from build123d import *

# Parameters (mm, degrees)
SKETCH1_R           = 47.625
BOSS_EXTRUDE1_DEPTH = 19.05
CUT_EXTRUDE1_DEPTH  = 70.9941694
CIRPATTERN1_COUNT   = 10
CUT_EXTRUDE2_DEPTH  = 15.24
SKETCH5_R           = 4.064
CUT_EXTRUDE3_DEPTH  = 70.054607739
CUT_EXTRUDE4_DEPTH  = 70.9941694


with BuildPart() as part:
    # Sketch1 → Boss-Extrude1 (new body)
    with BuildSketch(Plane(origin=(0, 0, 0), x_dir=(1, 0, 0), z_dir=(0, 1, 0))):
        with Locations(Location((0, 0, 0), (0, 0, 90))):
            Circle(SKETCH1_R)
    extrude(amount=BOSS_EXTRUDE1_DEPTH)

    # Sketch3 → Cut-Extrude1 (cut, symmetric)
    with BuildSketch(Plane(origin=(0, 19.05, 0), x_dir=(1, 0, 0), z_dir=(0, 1, 0))):
        with BuildLine():
            Line((0, 47.625), (0, 34.925))
            ThreePointArc((0, 34.925), (5.463473692, 34.495015295), (10.792418529, 33.215648832))
            Line((10.792418529, 33.215648832), (14.716934357, 45.294066589))
            ThreePointArc((14.716934357, 45.294066589), (7.450191398, 47.038657221), (0, 47.625))
        make_face()
    cut_extrude1 = extrude(amount=CUT_EXTRUDE1_DEPTH, both=True, mode=Mode.SUBTRACT)

    # CirPattern1: Cut-Extrude1 ×10 about axis
    cirpattern1_axis = Axis((0, 0, 0), (0, 1, 0))
    for i in range(1, CIRPATTERN1_COUNT):
        add(cut_extrude1.rotate(cirpattern1_axis, i * 360 / CIRPATTERN1_COUNT), mode=Mode.SUBTRACT)

    # Sketch4 → Cut-Extrude2 (cut)
    with BuildSketch(Plane(origin=(0, 19.05, 0), x_dir=(1, 0, 0), z_dir=(0, 1, 0))):
        Polygon((-3.519527241, 6.096), (3.519527241, 6.096), (7.039054482, 0), (3.519527241, -6.096), (-3.519527241, -6.096), (-7.039054482, 0), align=None)
    extrude(amount=-CUT_EXTRUDE2_DEPTH, mode=Mode.SUBTRACT)

    # Sketch5 → Cut-Extrude3 (cut, through all)
    with BuildSketch(Plane(origin=(0, 3.81, 0), x_dir=(1, 0, 0), z_dir=(0, 1, 0))):
        with Locations(Location((0, 0, 0), (0, 0, 270))):
            Circle(SKETCH5_R)
    extrude(amount=-CUT_EXTRUDE3_DEPTH, mode=Mode.SUBTRACT)

    # Sketch6 → Cut-Extrude4 (cut, through all)
    with BuildSketch(Plane(origin=(0, 19.05, 0), x_dir=(1, 0, 0), z_dir=(0, 1, 0))):
        with BuildLine():
            ThreePointArc((-11.225320151, 11.225320151), (-6.075099489, 14.666587579), (0, 15.875))
            Line((0, 15.875), (0, 27.94))
            ThreePointArc((0, 27.94), (-10.6921751, 25.813194138), (-19.756563466, 19.756563466))
            Line((-19.756563466, 19.756563466), (-11.225320151, 11.225320151))
        make_face()
        with BuildLine():
            Line((19.756563466, 19.756563466), (11.225320151, 11.225320151))
            ThreePointArc((11.225320151, 11.225320151), (14.666587579, 6.075099489), (15.875, 0))
            Line((15.875, 0), (27.94, 0))
            ThreePointArc((27.94, 0), (25.813194138, 10.6921751), (19.756563466, 19.756563466))
        make_face()
        with BuildLine():
            Line((19.756563466, -19.756563466), (11.225320151, -11.225320151))
            ThreePointArc((11.225320151, -11.225320151), (6.075099489, -14.666587579), (0, -15.875))
            Line((0, -15.875), (0, -27.94))
            ThreePointArc((0, -27.94), (10.6921751, -25.813194138), (19.756563466, -19.756563466))
        make_face()
        with BuildLine():
            Line((-19.756563466, -19.756563466), (-11.225320151, -11.225320151))
            ThreePointArc((-11.225320151, -11.225320151), (-14.666587579, -6.075099489), (-15.875, 0))
            Line((-15.875, 0), (-27.94, 0))
            ThreePointArc((-27.94, 0), (-25.813194138, -10.6921751), (-19.756563466, -19.756563466))
        make_face()
    extrude(amount=-CUT_EXTRUDE4_DEPTH, mode=Mode.SUBTRACT)


solid = part.part
Geometry: final body of the model. Coordinates: model frame, mm. A direction names the side the tool comes from. Coordinates: 2 decimals unless noted, no trailing zeros. Order: outer loops, then holes, each group sorted by start corner. A loop starts at its lowest first (then second) coordinate and runs counter-clockwise, first axis right, second up.
1) Section A-A (x = -17). Return loops of the section in (y, z).
Result sheet:
outline: (0, -30.51) - (19.05, -30.51) - (19.05, -22.17) - (0, -22.17) - close; (0, -17) - (19.05, -17) - (19.05, 0) - (0, 0) - close; (0, 17) - (19.05, 17) - (19.05, 44.49) - (0, 44.49) - close
2) Section C-C (z = -9.5). Return loops of the section in (x, y).
Result sheet:
outline: (-46.67, 0) - (12.72, 0) - (12.72, 19.05) - (-46.67, 19.05) - close; (26.28, 0) - (33.61, 0) - (33.61, 19.05) - (26.28, 19.05) - close
3) Section B-B (z = -25.5). Return loops of the section in (x, y).
Result sheet:
outline: (-35.1, 0) - (-11.42, 0) - (-11.42, 19.05) - (-35.1, 19.05) - close; (0, 0) - (23.86, 0) - (23.86, 19.05) - (0, 19.05) - close; (35.1, 0) - (40.22, 0) - (40.22, 19.05) - (35.1, 19.05) - close
4) Set-up query: faces 5 (the flat face through (0, 12, 6.096)), 6 (the cylindrical face through (6.16, 9.66, 14.63)), 7 (the flat face through (-24.31, 9.66, 33.46)). Return all of +Z, -Z, +X, -X, +Y, -Y with unobstructed straight access to the full face (end or side cutting, diameter ignored); none if empty.
Result sheet:
face 5: +Y
face 6: +Y, -Y
face 7: -X, +Y, -Y
5) First-contact query: P1, Ø10, axis at x = -9, y = 4, coming from the -Z side; P2, Ø6.5, axis at x = 38.5, y = 7, coming from the -Z side; P3, Ø4, axis at y = 11, z = -39, coming from the +X side; P4, Ø5.5, axis at x = 1.5, y = 10, coming from the -Z side (3 decimals). Flat tips, straight axial feed; report the tip coordinate or a pass-through.
Result sheet:
P1: stops at z = -47.46
P2: stops at z = -27.99
P3: stops at x = 27.99
P4: stops at z = -47.625
6) Section D-D (y = 8.25). Give the number of separate pieces and of enclosed holes in the cut face, then the cut area to 3 significant figures.
Result sheet:
separate pieces: 1
enclosed holes: 5
area: 4,520 mm2
7) Draft query along Z for faces 1 (the flat face through (10, 0, 1)), 2 (the cylindrical face through (-5.388, 9.658, 34.507)), 3 (the flat face through (33.32, 9.66, 24.21)), 4 (the cylindrical face through (14.63, 9.66, -6.16)). Return one class per face: released by +Z, released by -Z, zero draft, split by the parting line, or undercut.
Result sheet:
face 1: zero draft
face 2: released by +Z
face 3: undercut
face 4: undercut
8) Ray query, probe 1 along X at (y, z) = (15, 17.5); probe 2 along Z at (x, y) = (21, 16); probe 3 along X at (y, z) = (16.25, -42). Return the intervals inside material, ascending.
Result sheet:
probe 1: x = -44.29 to -21.78, -17.5 to 0, 17.5 to 30.22
probe 2: z = -42.75 to -28.9, -27.91 to -18.43, 0 to 28.9
probe 3: x = -13.65 to 0, 13.65 to 22.45
